Model file for the job. Use its own axes, mm. A direction names the side the tool comes from. Round coordinates to 2 decimals unless told otherwise and drop trailing zeros. Order: outer loops, then holes, each group sorted by start corner. A loop starts at its lowest first (then second) coordinate and runs counter-clockwise, first axis right, second up. Notation, with made-up numbers: (66.25, 36) - (112.25, 36) arc R23 cw to (112.25, 68) - close; hole circle Ø1 at (30, 27.5). An arc over 180 degrees is marked (long way). Use one line per item in the form item = value.
from build123d import *

# Parameters (mm, degrees)
SKETCH1_R                                            = 60
SKETCH1_R_2                                          = 33
BOSS_EXTRUDE1_DEPTH                                  = 5
SKETCH2_R                                            = 49.5
SKETCH2_R_2                                          = 42.6
BOSS_EXTRUDE2_DEPTH                                  = 10
SKETCH3_R                                            = 1.7
CUT_EXTRUDE1_DEPTH                                   = 5
SKETCH5_R                                            = 1.5
CUT_EXTRUDE2_DEPTH                                   = 5
CBORE_FOR_M5_HEX_SOCKET_THIN_HEAD_CAP_SC_D           = 3
CBORE_FOR_M5_HEX_SOCKET_THIN_HEAD_CAP_SC_CBORE_D     = 5.2
CBORE_FOR_M5_HEX_SOCKET_THIN_HEAD_CAP_SC_CBORE_DEPTH = 1.7


with BuildPart() as part:
    # Sketch1 → Boss-Extrude1 (new body)
    with BuildSketch(Plane.XY):
        Circle(SKETCH1_R)
        Circle(SKETCH1_R_2, mode=Mode.SUBTRACT)
    extrude(amount=BOSS_EXTRUDE1_DEPTH)

    # Sketch2 → Boss-Extrude2 (add)
    with BuildSketch(Plane(origin=(0, 0, 0), x_dir=(-1, 0, 0), z_dir=(0, 0, -1))):
        Circle(SKETCH2_R)
        Circle(SKETCH2_R_2, mode=Mode.SUBTRACT)
    extrude(amount=BOSS_EXTRUDE2_DEPTH)

    # Sketch3 → Cut-Extrude1 (cut)
    with BuildSketch(Plane(origin=(0, 0, -10), x_dir=(-1, 0, 0), z_dir=(0, 0, -1))):
        with Locations((0, 45)):
            Circle(SKETCH3_R)
        with Locations((5.52997308, 44.658922935)):
            Circle(SKETCH3_R)
        with Locations((10.976117405, 43.640862122)):
            Circle(SKETCH3_R)
        with Locations((16.255874978, 41.961250323)):
            Circle(SKETCH3_R)
        with Locations((21.289210058, 39.645548743)):
            Circle(SKETCH3_R)
        with Locations((25.999822413, 36.728861056)):
            Circle(SKETCH3_R)
        with Locations((30.316303964, 33.255401275)):
            Circle(SKETCH3_R)
        with Locations((34.173221249, 29.277823509)):
            Circle(SKETCH3_R)
        with Locations((37.512107335, 24.856423783)):
            Circle(SKETCH3_R)
        with Locations((40.282348111, 20.05822601)):
            Circle(SKETCH3_R)
        with Locations((42.441949551, 14.955965977)):
            Circle(SKETCH3_R)
        with Locations((43.958174299, 9.626988744)):
            Circle(SKETCH3_R)
        with Locations((44.808037933, 4.152076176)):
            Circle(SKETCH3_R)
        with Locations((44.978657387, -1.385777635)):
            Circle(SKETCH3_R)
        with Locations((44.467446244, -6.90262447)):
            Circle(SKETCH3_R)
        with Locations((43.282153943, -12.314834553)):
            Circle(SKETCH3_R)
        with Locations((41.440748308, -17.540364298)):
            Circle(SKETCH3_R)
        with Locations((38.97114317, -22.5)):
            Circle(SKETCH3_R)
        with Locations((35.910775228, -27.118558637)):
            Circle(SKETCH3_R)
        with Locations((32.306036538, -31.326027568)):
            Circle(SKETCH3_R)
        with Locations((28.211571265, -35.058625854)):
            Circle(SKETCH3_R)
        with Locations((23.689447329, -38.259771108)):
            Circle(SKETCH3_R)
        with Locations((18.80821552, -40.880937232)):
            Circle(SKETCH3_R)
        with Locations((13.641870335, -42.882390019)):
            Circle(SKETCH3_R)
        with Locations((8.268728302, -44.233789486)):
            Circle(SKETCH3_R)
        with Locations((2.770240776, -44.914649793)):
            Circle(SKETCH3_R)
        with Locations((-2.770240776, -44.914649793)):
            Circle(SKETCH3_R)
        with Locations((-8.268728302, -44.233789486)):
            Circle(SKETCH3_R)
        with Locations((-13.641870335, -42.882390019)):
            Circle(SKETCH3_R)
        with Locations((-18.80821552, -40.880937232)):
            Circle(SKETCH3_R)
        with Locations((-23.689447329, -38.259771108)):
            Circle(SKETCH3_R)
        with Locations((-28.211571265, -35.058625854)):
            Circle(SKETCH3_R)
        with Locations((-32.306036538, -31.326027568)):
            Circle(SKETCH3_R)
        with Locations((-35.910775228, -27.118558637)):
            Circle(SKETCH3_R)
        with Locations((-38.97114317, -22.5)):
            Circle(SKETCH3_R)
        with Locations((-41.440748308, -17.540364298)):
            Circle(SKETCH3_R)
        with Locations((-43.282153943, -12.314834553)):
            Circle(SKETCH3_R)
        with Locations((-44.467446244, -6.90262447)):
            Circle(SKETCH3_R)
        with Locations((-44.978657387, -1.385777635)):
            Circle(SKETCH3_R)
        with Locations((-44.808037933, 4.152076176)):
            Circle(SKETCH3_R)
        with Locations((-43.958174299, 9.626988744)):
            Circle(SKETCH3_R)
        with Locations((-42.441949551, 14.955965977)):
            Circle(SKETCH3_R)
        with Locations((-40.282348111, 20.05822601)):
            Circle(SKETCH3_R)
        with Locations((-37.512107335, 24.856423783)):
            Circle(SKETCH3_R)
        with Locations((-34.173221249, 29.277823509)):
            Circle(SKETCH3_R)
        with Locations((-30.316303964, 33.255401275)):
            Circle(SKETCH3_R)
        with Locations((-25.999822413, 36.728861056)):
            Circle(SKETCH3_R)
        with Locations((-21.289210058, 39.645548743)):
            Circle(SKETCH3_R)
        with Locations((-16.255874978, 41.961250323)):
            Circle(SKETCH3_R)
        with Locations((-10.976117405, 43.640862122)):
            Circle(SKETCH3_R)
        with Locations((-5.52997308, 44.658922935)):
            Circle(SKETCH3_R)
    extrude(amount=-CUT_EXTRUDE1_DEPTH, mode=Mode.SUBTRACT)

    # Sketch5 → Cut-Extrude2 (cut)
    with BuildSketch(Plane.XY.offset(5)):
        with Locations((0, 55)):
            Circle(SKETCH5_R)
        with Locations((47.631397208, 27.5)):
            Circle(SKETCH5_R)
        with Locations((47.631397208, -27.5)):
            Circle(SKETCH5_R)
        with Locations((0, -55)):
            Circle(SKETCH5_R)
        with Locations((-47.631397208, -27.5)):
            Circle(SKETCH5_R)
        with Locations((-47.631397208, 27.5)):
            Circle(SKETCH5_R)
    extrude(amount=-CUT_EXTRUDE2_DEPTH, mode=Mode.SUBTRACT)

    # CBORE for M5 Hex Socket Thin Head Cap Screw4 (through all)
    with Locations(Plane(origin=(-47.631397208, 27.5, 5), x_dir=(1, 0, 0), z_dir=(0, 0, 1))):
        with Locations((0, 0), (47.631397208, 27.5), (95.262794416, 0), (95.262794416, -55), (47.631397208, -82.5), (0, -55)):
            CounterBoreHole(CBORE_FOR_M5_HEX_SOCKET_THIN_HEAD_CAP_SC_D / 2, CBORE_FOR_M5_HEX_SOCKET_THIN_HEAD_CAP_SC_CBORE_D / 2, CBORE_FOR_M5_HEX_SOCKET_THIN_HEAD_CAP_SC_CBORE_DEPTH)


solid = part.part
(1) Slice it at B-B on y = -22.5. Give the cut face in (x, z), then the cut area to 3 significant figures.
Report:
outline = (-55.62, 0) - (-44.09, 0) - (-44.09, -10) - (-40.67, -10) - (-40.67, -5) - (-37.27, -5) - (-37.27, -10) - (-36.17, -10) - (-36.17, 0) - (-24.14, 0) - (-24.14, 5) - (-55.62, 5) - close; (24.14, 0) - (36.17, 0) - (36.17, -10) - (37.27, -10) - (37.27, -5) - (40.67, -5) - (40.67, -10) - (44.09, -10) - (44.09, 0) - (55.62, 0) - (55.62, 5) - (24.14, 5) - close
area = 439 mm2
(2) Slice it at C-C on z = -7.75. Count the separate pieces of the cut face and the enclosed holes in it, then the cut area to 3 significant figures.
Report:
separate_pieces = 1
enclosed_holes = 52
area = 1,530 mm2
(3) Probe probe 1 along Y at (x, z) = (0, 1.5); probe 2 along Y at (x, z) = (-25, -8); probe 3 along Y at (x, z) = (21, -9). List the from-to ranges inside material, lowest first. Write a range as [from, to].
Report:
probe_1 = [-60, -56.5], [-53.5, -33], [33, 53.5], [56.5, 60]
probe_2 = [-42.72, -39.34], [-37.18, -34.49], [34.49, 35.35], [38.1, 42.72]
probe_3 = [-44.82, -37.06], [37.06, 37.97], [41.32, 44.82]
(4) Pull direction X, two halves, no side cores. Call faces 3 (the face through (-0.56, 52.46, 4.16)), 4 (the face through (6.44, 49.08, -4.93)), 5 (the face through (18.024, -42.389, -7.535)): released by +X, released by -X, zero draft, split by the parting line, or undercut.
Report:
face_3 = undercut
face_4 = split by the parting line
face_5 = undercut
(5) Pin check, flat tips, straight feed: pin 1 (1.5 mm diameter, centred on y = 2.5, z = -6.5, fed in from +X); pin 2 (1.5 mm diameter, centred on y = -4, z = -5.5, fed in from -X); pin 3 (3 mm diameter, centred on x = 23.69, y = -38.26, fed in from -Z). Stop position of each tip, or through.
Report:
pin_1 = 49.47
pin_2 = -49.39
pin_3 = -5
(6) Tool access for faces 1 (the face through (49.062, -27.049, 1.673)), 2 (the face through (0, 45, -5)): list every direction of +Z, -Z, +X, -X, +Y, -Y with a clear straight run to the whole face (end or side of a thin tool).
Report:
face_1 = +Z, -Z
face_2 = -Z
(7) Slice it at A-A on y = 55. Give the cut face in (x, z), then the cut area to 3 significant figures.
Report:
outline = (-23.98, 0) - (-1.5, 0) - (-1.5, 3.3) - (-2.6, 3.3) - (-2.6, 5) - (-23.98, 5) - close; (1.5, 0) - (23.98, 0) - (23.98, 5) - (2.6, 5) - (2.6, 3.3) - (1.5, 3.3) - close
area = 221 mm2
